For this review, take the finished solid that the model builds, in its own axes (mm). Give positions to 0.01 mm unless a question says otherwise; leave off trailing zeros. Write each loop counter-clockwise with the first axis right and the second up, starting at its lowest first coordinate (ties: lowest second). Pieces come first, ordered by that corner, then holes. Notation, with made-up numbers: M 66.5,68.25 L 80.5,68.25 A8 cw 80.5,80.25 Z; hole C 85.5,-5 d2. An arc over 180 degrees is marked long. One line per item, written item: value. Start each with the question number.
Item 1: Consider section C-C, the plane x = 21. Give the number of separate pieces and of enclosed holes in the cut face, and give its area (3 significant figures).
Item 2: Consider section A-A, the plane z = 0. Write out the cut boundary in (x, y) (3 decimals), and give its area (3 significant figures).
Item 3: Consider section B-B, the plane y = -10. Write out the cut boundary in (x, z) (3 decimals).
Item 4: To check wall thickness, follow probe 1 along Y at (x, z) = (28.5, -7.25); probe 2 along Z at (x, y) = (155, 0.5); probe 3 along Y at (x, z) = (44, -3) (3 decimals). State the ranges of each line that lie inside material, in increasing order.
Item 5: Clearance check with a flat-ended pin moving along its axis: pin 1 Ø2 at (x, z) = (111.5, 1) entering from +Y (3 decimals). State where the tip first meets the part, or that it passes through.
```python
from build123d import *

# Parameters (mm, degrees)
F0_R     = 2
F1_DEPTH = 200


with BuildPart() as f1:
    # F0 (on Right) → F1 (new body)
    with BuildSketch(Plane.YZ):
        Polygon((6.935, 10), (0, 10), (-6.935, 10), (-6.935, 8.05), (-4, 8.05), (-4, 6.999239), (-7.074239, 3.925), (-13.005761, 3.925), (-16.08, 6.999239), (-16.08, 8.05), (-13.12, 8.05), (-13.12, 10), (-20, 10), (-20, 3.12), (-18.05, 3.12), (-18.05, 6.08), (-16.999239, 6.08), (-13.925, 3.005761), (-13.925, 0), (-13.925, -3.005761), (-16.999239, -6.08), (-18.05, -6.08), (-18.05, -3.12), (-20, -3.12), (-20, -10), (-13.12, -10), (-13.12, -8.05), (-16.08, -8.05), (-16.08, -6.999239), (-13.005761, -3.925), (-7.074239, -3.925), (-4, -6.999239), (-4, -8.05), (-6.935, -8.05), (-6.935, -10), (0, -10), (6.935, -10), (6.935, -8.05), (4, -8.05), (4, -6.999239), (7.074239, -3.925), (13.005761, -3.925), (16.08, -6.999239), (16.08, -8.05), (13.12, -8.05), (13.12, -10), (20, -10), (20, -3.12), (18.05, -3.12), (18.05, -6.08), (16.999239, -6.08), (13.925, -3.005761), (13.925, 0), (13.925, 3.005761), (16.999239, 6.08), (18.05, 6.08), (18.05, 3.12), (20, 3.12), (20, 10), (13.12, 10), (13.12, 8.05), (16.08, 8.05), (16.08, 6.999239), (13.005761, 3.925), (7.074239, 3.925), (4, 6.999239), (4, 8.05), (6.935, 8.05), align=None)
        with Locations((-10, 0)):
            Circle(F0_R, mode=Mode.SUBTRACT)
        Polygon((-2.161522, 8.05), (0, 8.05), (2.161522, 8.05), (2.161522, 6.999239), (6.075, 3.085761), (6.075, 0), (6.075, -3.085761), (2.161522, -6.999239), (2.161522, -8.05), (0, -8.05), (-2.161522, -8.05), (-2.161522, -6.999239), (-6.075, -3.085761), (-6.075, 0), (-6.075, 3.085761), (-2.161522, 6.999239), align=None, mode=Mode.SUBTRACT)
        with Locations((10, 0)):
            Circle(F0_R, mode=Mode.SUBTRACT)
    extrude(amount=F1_DEPTH)


solid = f1.part
```
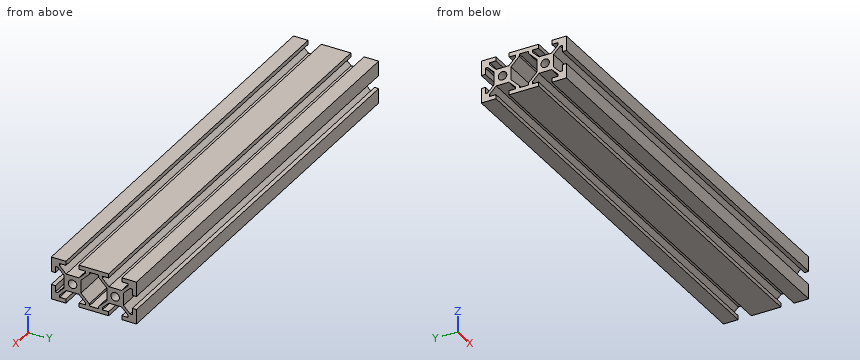
Model answer:
1. separate pieces: 1
1. enclosed holes: 3
1. area: 311 mm2
2. outline: M 0,-13.925 L 200,-13.925 L 200,-12 L 0,-12 Z; M 0,-8 L 200,-8 L 200,-6.075 L 0,-6.075 Z; M 0,6.075 L 200,6.075 L 200,8 L 0,8 Z; M 0,12 L 200,12 L 200,13.925 L 0,13.925 Z
2. area: 1,540 mm2
3. outline: M 0,-3.925 L 200,-3.925 L 200,-2 L 0,-2 Z; M 0,2 L 200,2 L 200,3.925 L 0,3.925 Z
4. probe 1: y = -20 to -16.08, -4 to -2.16, 2.16 to 4, 16.08 to 20
4. probe 2: z = -10 to -8.05, 8.05 to 10
4. probe 3: y = -13.925 to -6.075, 6.075 to 13.925
5. pin 1: stops at y = 13.925
